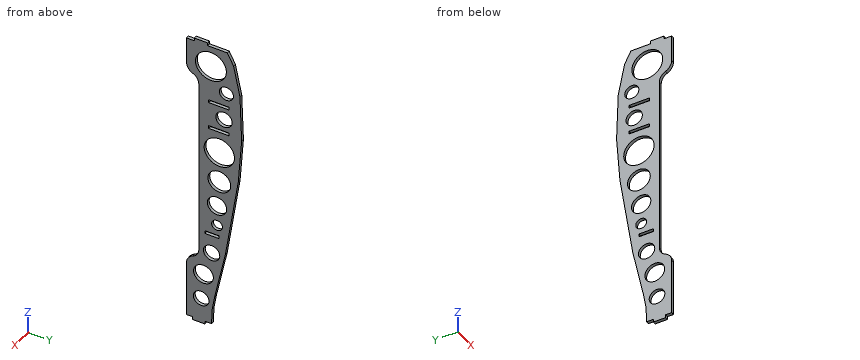
from build123d import *

# Parameters (mm, degrees)
BOSS_EXTRUDE1_DEPTH = 3
CUT_EXTRUDE1_DEPTH  = 3
FILLET1_R           = 10
SKETCH3_R           = 8
CUT_EXTRUDE2_DEPTH  = 3
SKETCH5_W           = 3
SKETCH5_H           = 13
SKETCH5_H_2         = 12
BOSS_EXTRUDE2_DEPTH = 3
SKETCH6_R           = 15.147681316
SKETCH6_R_2         = 6.940415837
SKETCH6_R_3         = 14.88620922
SKETCH6_R_4         = 11.185928508
SKETCH6_R_5         = 9.478125157
SKETCH6_R_6         = 5.324718802
SKETCH6_R_7         = 8.008616256
SKETCH6_R_8         = 9.712526273
SKETCH6_R_9         = 7.687216176
SKETCH6_W           = 3
SKETCH6_H           = 20
SKETCH6_H_2         = 14
CUT_EXTRUDE3_DEPTH  = 10


with BuildPart() as part:
    # Sketch1 → Boss-Extrude1 (new body)
    with BuildSketch(Plane(origin=(0, 0, 0), x_dir=(0, 0, -1), z_dir=(1, 0, 0))):
        Polygon((0, 0), (11.910798094, 6.158004928), (42.739414765, 12.383521095), (90.106781804, 14.033136775), (135.887385092, 10.713704644), (219.287488067, -1.876713431), (270.057015241, -12.532639482), (283.823146281, -14.792882614), (299.988096251, -15.517362165), (299.988096251, -40), (0, -40), align=None)
    extrude(amount=BOSS_EXTRUDE1_DEPTH)

    # Sketch2 → Cut-Extrude1 (cut)
    with BuildSketch(Plane(origin=(3, 0, 0), x_dir=(0, 0, -1), z_dir=(1, 0, 0))):
        with BuildLine():
            Line((35, -40), (35, -38))
            ThreePointArc((35, -38), (37.928932188, -30.928932188), (45, -28))
            Line((45, -28), (225, -28))
            ThreePointArc((225, -28), (232.071067812, -30.928932188), (235, -38))
            Line((235, -38), (235, -40))
            Line((235, -40), (35, -40))
        make_face()
    extrude(amount=-CUT_EXTRUDE1_DEPTH, mode=Mode.SUBTRACT)

    # Fillet1
    fillet1_edges = [part.edges().sort_by_distance(p)[0] for p in [
        (1.5, -40, -235),
        (1.5, -40, -35),
    ]]
    fillet(fillet1_edges, radius=FILLET1_R)

    # Sketch3 → Cut-Extrude2 (cut)
    with BuildSketch(Plane(origin=(3, 0, 0), x_dir=(0, 0, -1), z_dir=(1, 0, 0))):
        with Locations((73.81, -3.27)):
            Circle(SKETCH3_R)
    extrude(amount=-CUT_EXTRUDE2_DEPTH, mode=Mode.SUBTRACT)

    # Sketch5 → Boss-Extrude2 (add)
    with BuildSketch(Plane(origin=(3, 0, 0), x_dir=(0, 0, -1), z_dir=(1, 0, 0))):
        with Locations((-1.5, -25.8)):
            Rectangle(SKETCH5_W, SKETCH5_H)
        with Locations((301.488096251, -28.017362165)):
            Rectangle(SKETCH5_W, SKETCH5_H_2)
    extrude(amount=-BOSS_EXTRUDE2_DEPTH)

    # Sketch6 → Cut-Extrude3 (cut)
    with BuildSketch(Plane(origin=(3, 0, 0), x_dir=(0, 0, -1), z_dir=(1, 0, 0))):
        with Locations((21.242347481, -16.071768518)):
            Circle(SKETCH6_R)
        with Locations((44.884098964, -0.924087202)):
            Circle(SKETCH6_R_2)
        with Locations((111.33658962, -7.864503039)):
            Circle(SKETCH6_R_3)
        with Locations((143.071913682, -7.864503039)):
            Circle(SKETCH6_R_4)
        with Locations((170.121485199, -10.108083459)):
            Circle(SKETCH6_R_5)
        with Locations((191.207371657, -10.108083459)):
            Circle(SKETCH6_R_6)
        with Locations((223.368673224, -15.432802262)):
            Circle(SKETCH6_R_7)
        with Locations((249.566289732, -23.441418517)):
            Circle(SKETCH6_R_8)
        with Locations((276.615861249, -25.656262362)):
            Circle(SKETCH6_R_9)
        with Locations((59.81, -8.27)):
            Rectangle(SKETCH6_W, SKETCH6_H)
        with Locations((87.81, -8.27)):
            Rectangle(SKETCH6_W, SKETCH6_H)
        with Locations((203.245, -15)):
            Rectangle(SKETCH6_W, SKETCH6_H_2)
    extrude(amount=-CUT_EXTRUDE3_DEPTH, mode=Mode.SUBTRACT)


solid = part.part
Input: part model. Units: mm. Frame: model coordinates. Give positions to 0.01 mm unless a question says otherwise; leave off trailing zeros. Loops run counter-clockwise (first coordinate to the right, second up) from the corner with the lowest first, then second, coordinate; pieces in that order, holes last. Notation, with made-up numbers: (54.5, 79.25) - (103.5, 79.25) arc R18 ccw to (103.5, 96.25) - close; hole circle Ø6 at (3.25, 3.25). An arc over 180 degrees is marked (long way). Use CSV: the item, a comma, the result in double quotes. Start each with the question number.
Item 1: Section C-C on z = -73.81. Return loops of the section in (x, y), then the cut area to 3 significant figures.
Item 2: Section B-B on x = 2.3. State how many separate pieces and enclosed holes the cut face has, then the cut area to 3 significant figures.
Item 3: Section D-D on z = -212.5. Return loops of the section in (x, y), then the cut area to 3 significant figures.
Item 4: Line query: line 1 (Y direction, x = 2.6, z = -31.5); line 2 (Y direction, x = 1.35, z = -136.5); line 3 (Z direction, x = 2.45, y = -34.5). Output: solid intervals per line, ascending.
Item 5: Contact query for flat-ended pins moving along their axis: P1, Ø1, axis at x = 0.5, z = -30, coming from the -Y side; P2, Ø1.5, axis at x = 1, z = -222.5, coming from the -Y side; P3, Ø14.5, axis at y = -15.43, z = -223.37, coming from the -X side; P4, Ø17.5, axis at y = -25.66, z = -276.62, coming from the -X side. Output: stop coordinate, or through.
Item 6: Section A-A on z = -142. Return loops of the section in (x, y), then the cut area to 3 significant figures.
Ans:
1,outline,"(0, -28) - (3, -28) - (3, -11.27) - (0, -11.27) - close; (0, 4.73) - (3, 4.73) - (3, 13.47) - (0, 13.47) - close"
1,area,"76.4 mm2"
2,separate pieces,"1"
2,enclosed holes,"13"
2,area,"7,400 mm2"
3,outline,"(0, -28) - (3, -28) - (3, -0.85) - (0, -0.85) - close"
3,area,"81.4 mm2"
4,line 1,"y = -38.76 to -27.22, -4.93 to 10.11"
4,line 2,"y = -28 to -16.92, 1.19 to 10.62"
4,line 3,"z = -299.99 to -234.4, -35.6 to 0"
5,P1,"stops at y = -39.59"
5,P2,"stops at y = -28"
5,P3,"passes through"
5,P4,"stops at x = 0"
6,outline,"(0, -28) - (3, -28) - (3, -19) - (0, -19) - close; (0, 3.27) - (3, 3.27) - (3, 9.79) - (0, 9.79) - close"
6,area,"46.6 mm2"
